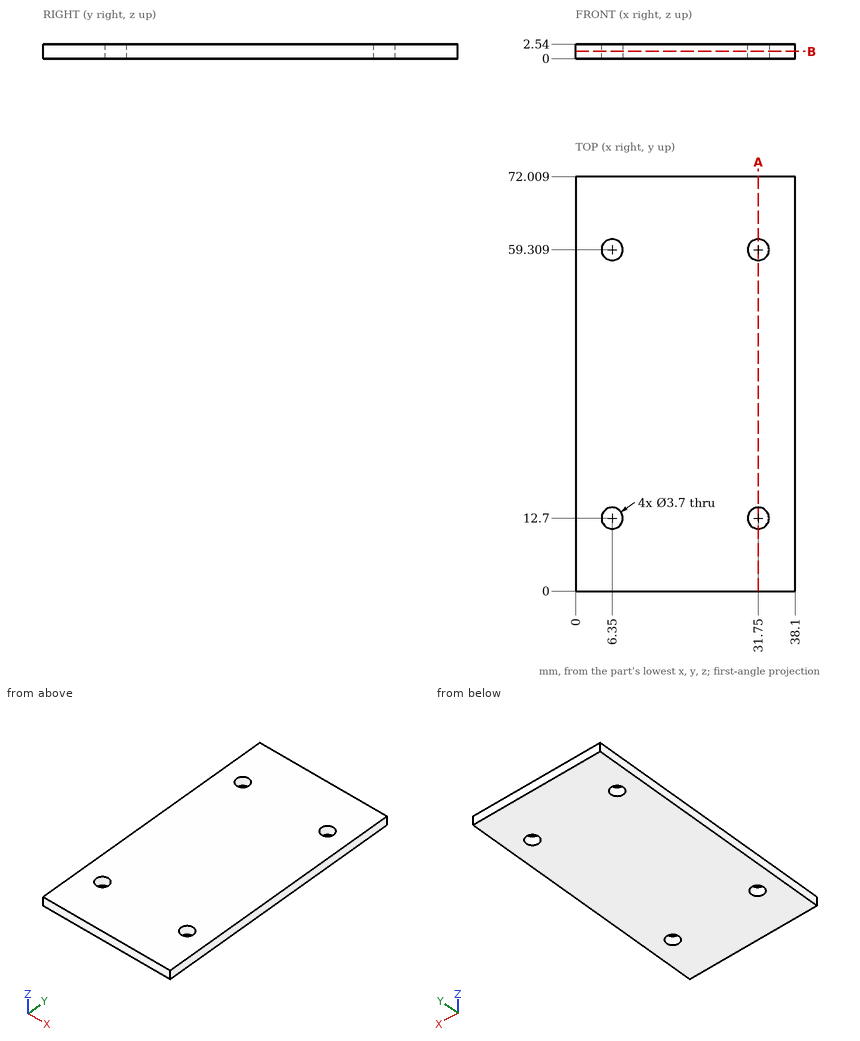
Answer from the drawing. Dimensions are ordinates in mm from the lowest x, y and z of the part. Give positions to 0.01 mm unless a question says otherwise; leave off trailing zeros. Order: outer loops, then holes, each group sorted by start corner. A loop starts at its lowest first (then second) coordinate and runs counter-clockwise, first axis right, second up. Notation, with made-up numbers: (86, 75) - (92, 75) arc R24 cw to (92, 100) - close; hole circle Ø3 at (-12, 41.25). An arc over 180 degrees is marked (long way). Use one line per item in the form item = value.
1) This flat-tipped pin is pushed along its axis until it touches: pin 1 (3.5 mm diameter, centred on x = 6.35, y = 12.7, fed in from -Z). Where does it stop, or does it pass through?
Verdict:
pin_1 = through
2) Consider probe 1 along Y at (x, z) = (6.35, 0.9); probe 2 along X at (y, z) = (59.5, 0.35); probe 3 along X at (y, z) = (12, 1.15). Determine where each line is inside the solid, lowest interval first. Write a range as [from, to].
Verdict:
probe_1 = [0, 10.85], [14.55, 57.46], [61.16, 72.01]
probe_2 = [0, 4.51], [8.19, 29.91], [33.59, 38.1]
probe_3 = [0, 4.64], [8.06, 30.04], [33.46, 38.1]
3) Find section B-B on z = 1.25. Determine the outline of the cut face in (x, y).
Verdict:
outline = (0, 0) - (38.1, 0) - (38.1, 72.01) - (0, 72.01) - close; hole circle Ø3.7 at (6.35, 12.7); hole circle Ø3.7 at (6.35, 59.31); hole circle Ø3.7 at (31.75, 12.7); hole circle Ø3.7 at (31.75, 59.31)
4) Find section A-A on x = 31.75. Determine the outline of the cut face in (y, z), and give its area (3 significant figures).
Verdict:
outline = (0, 0) - (10.85, 0) - (10.85, 2.54) - (0, 2.54) - close; (14.55, 0) - (57.46, 0) - (57.46, 2.54) - (14.55, 2.54) - close; (61.16, 0) - (72.01, 0) - (72.01, 2.54) - (61.16, 2.54) - close
area = 164 mm^2
